Geometry: see drawing. Coordinates: mm, zero at the bounding-box minimum. A direction names the side the tool comes from. Coordinates: 2 decimals unless noted, no trailing zeros. Order: outer loops, then holes, each group sorted by start corner. A loop starts at its lowest first (then second) coordinate and runs counter-clockwise, first axis right, second up.
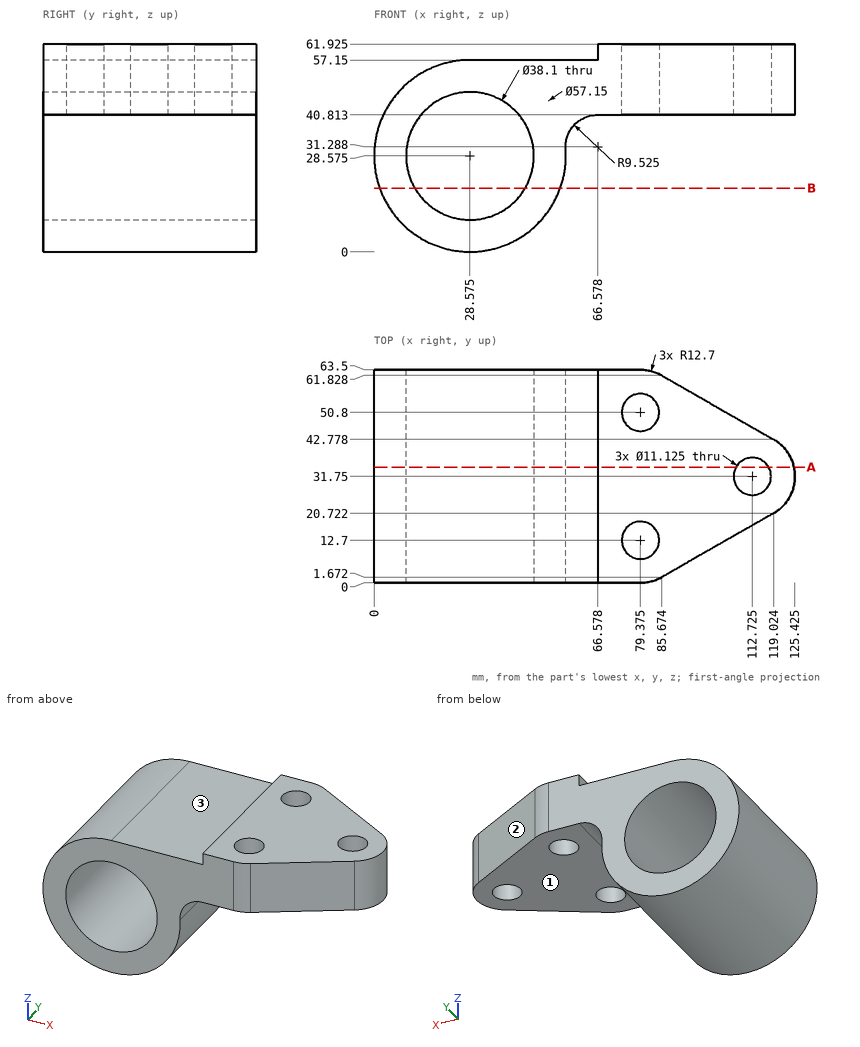
Q1. Pin query (flat end, axial travel): P1, Ø6.5, axis at x = 112.73, y = 31.75, coming from the -Z side; P2, Ø10, axis at x = 48.5, z = 7, coming from the -Y side; P3, Ø2, axis at y = 35.5, z = 54.5, coming from the +X side; P4, Ø1.4, axis at y = 31.5, z = 59.5, coming from the -X side. Return the tip coordinate at first contact, or that it passes through.
Solutions:
P1: passes through
P2: stops at y = 0
P3: stops at x = 125.12
P4: stops at x = 66.58
Q2. Section query A-A on y = 34.5. Give the number of separate pieces and of enclosed holes in the cut face.
Solutions:
separate pieces: 2
enclosed holes: 1
Q3. Material intervals for line 1 along Y through (x, z) = (78.5, 56); line 2 along Z through (x, y) = (23, 22.5); line 3 along Z through (x, y) = (27.5, 22) (1 decimal), sorted ascending.
Solutions:
line 1: y = 0 to 7.21, 18.19 to 45.31, 56.29 to 63.5
line 2: z = 0.55 to 10.36, 46.79 to 56.6
line 3: z = 0 to 9.6, 47.6 to 57.1
Q4. Section query B-B on z = 19. Output: boundary loops of the cut face in (x, y).
Solutions:
outline: (1.65, 0) - (12.11, 0) - (12.11, 63.5) - (1.65, 63.5) - close; (45.04, 0) - (55.5, 0) - (55.5, 63.5) - (45.04, 63.5) - close
Q5. Set-up query: the marked faces 1, 2 and 3. Return all of +Z, -Z, +X, -X, +Y, -Y with unobstructed straight access to the full face (end or side cutting, diameter ignored); none if empty.
Solutions:
face 1: -Z, +X, +Y, -Y
face 2: +Z, -Z, +X, +Y
face 3: +Z, -X, +Y, -Y
